CAD build for the part. Positions are in the model's coordinates, mm. A direction names the side the tool comes from. Coordinates: 2 decimals unless noted, no trailing zeros. Loops run counter-clockwise (first coordinate to the right, second up) from the corner with the lowest first, then second, coordinate; pieces in that order, holes last. Notation, with made-up numbers: (56.25, 60.25) -> (65.25, 60.25) arc R21 ccw to (65.25, 73.25) -> close; hole circle Ø7 at (-36.75, -27). An arc over 180 degrees is marked (long way). Write item = value, one per line. Start each with the question number.
(1) Drill centre lines: line 1 (Z direction, x = 3, y = 17.75); line 2 (Y direction, x = 16.5, z = 5); line 3 (Y direction, x = -14.5, z = 6.5). Where is each one in solid material? Low to high. Write a range as from..to.
(2) Band-saw the part on B-B (x = -17.5). Write the cut outline in (y, z), and give its area (3 significant figures).
(3) Pull direction X, two halves, no side cores. Call faces 1 (the face through (-21.5, 20, 0)), 2 (the face through (-16.49, 22.86, 7.39)), 3 (the face through (9, 18.8, 0)): +X half, -X half, draft (parallel to the pull), parting line (faces both ways), or undercut.
(4) Flat gauge pins, fed straight in: P1, Ø15, axis at x = -9.5, y = 5, coming from the -Z side; P2, Ø4, axis at x = 13.5, z = -9, coming from the -Y side; P3, Ø12, axis at x = 12, y = 21, coming from the -Z side; P4, Ø5, axis at y = 14, z = 5.5, coming from the +X side. Where does each tip first touch, or does it go through?
(5) Tool access for faces 4 (the face through (18.51, 22.86, 7.39)), 5 (the face through (-5, 9, -8.5)), 6 (the face through (-16.5, 9, 0)), 7 (the face through (-5, 9, 8)): list every direction of +Z, -Z, +X, -X, +Y, -Y with a clear straight run to the whole face (end or side of a thin tool).
(6) Band-saw the part on C-C (y = 14.75). Write the cut outline in (x, z), and give its area (3 significant figures).
(7) Band-saw the part on D-D (x = 1). Write the cut outline in (y, z).
(8) Band-saw the part on A-A (z = 8.5). Write the cut outline in (x, y), and give its area (3 significant figures).
```python
from build123d import *

# Parameters (mm, degrees)
P01_STANDOFF_START                = 20.4
SK_P01_STANDOFF_R                 = 1.5
P01_STANDOFF_DEPTH                = 5
P02_STANDOFF_START                = 20.4
SK_P02_STANDOFF_R                 = 1.5
P02_STANDOFF_DEPTH                = 5
P03_STANDOFF_START                = 20.4
SK_P03_STANDOFF_R                 = 1.5
P03_STANDOFF_DEPTH                = 5
P04_STANDOFF_START                = 20.4
SK_P04_STANDOFF_R                 = 1.5
P04_STANDOFF_DEPTH                = 5
P05_POLOLURCSWITCHWITHRELAY_START = 18.8
SK_P05_POLOLURCSWITCHWITHRELAY_W  = 43
SK_P05_POLOLURCSWITCHWITHRELAY_H  = 25
P05_POLOLURCSWITCHWITHRELAY_DEPTH = 1.6
SK_P06_RELAYG5LE_W                = 22.5
SK_P06_RELAYG5LE_H                = 16.5
P06_RELAYG5LE_DEPTH               = 18.8


with BuildPart() as part:
    # SK_P01_Standoff → P01_Standoff (new body)
    with BuildSketch(Plane(origin=(0, 0, 0), x_dir=(1, 0, 0), z_dir=(0, 1, 0)).offset(P01_STANDOFF_START)):
        with Locations(Location((-17.5, 8.5, 0), (0, 0, 270))):
            Circle(SK_P01_STANDOFF_R)
    extrude(amount=P01_STANDOFF_DEPTH)



with BuildPart() as body_2:
    # SK_P02_Standoff → P02_Standoff (new body)
    with BuildSketch(Plane(origin=(0, 0, 0), x_dir=(1, 0, 0), z_dir=(0, 1, 0)).offset(P02_STANDOFF_START)):
        with Locations(Location((-17.5, -8.5, 0), (0, 0, 270))):
            Circle(SK_P02_STANDOFF_R)
    extrude(amount=P02_STANDOFF_DEPTH)


with BuildPart() as body_3:
    # SK_P03_Standoff → P03_Standoff (new body)
    with BuildSketch(Plane(origin=(0, 0, 0), x_dir=(1, 0, 0), z_dir=(0, 1, 0)).offset(P03_STANDOFF_START)):
        with Locations(Location((17.5, 8.5, 0), (0, 0, 270))):
            Circle(SK_P03_STANDOFF_R)
    extrude(amount=P03_STANDOFF_DEPTH)


with BuildPart() as body_4:
    # SK_P04_Standoff → P04_Standoff (new body)
    with BuildSketch(Plane(origin=(0, 0, 0), x_dir=(1, 0, 0), z_dir=(0, 1, 0)).offset(P04_STANDOFF_START)):
        with Locations(Location((17.5, -8.5, 0), (0, 0, 270))):
            Circle(SK_P04_STANDOFF_R)
    extrude(amount=P04_STANDOFF_DEPTH)


with BuildPart() as part_1:
    add(part.part)

    add(body_2.part)  # P05_PololuRCswitchwithrelay merges body 2

    add(body_3.part)  # P05_PololuRCswitchwithrelay merges body 3

    add(body_4.part)  # P05_PololuRCswitchwithrelay merges body 4
    # SK_P05_PololuRCswitchwithrelay → P05_PololuRCswitchwithrelay (add)
    with BuildSketch(Plane(origin=(0, 0, 0), x_dir=(1, 0, 0), z_dir=(0, 1, 0)).offset(P05_POLOLURCSWITCHWITHRELAY_START)):
        Rectangle(SK_P05_POLOLURCSWITCHWITHRELAY_W, SK_P05_POLOLURCSWITCHWITHRELAY_H)
    extrude(amount=P05_POLOLURCSWITCHWITHRELAY_DEPTH)

    # SK_P06_RelayG5LE → P06_RelayG5LE (add)
    with BuildSketch(Plane(origin=(0, 0, 0), x_dir=(1, 0, 0), z_dir=(0, 1, 0))):
        with Locations((-5.25, 0.25)):
            Rectangle(SK_P06_RELAYG5LE_W, SK_P06_RELAYG5LE_H)
    extrude(amount=P06_RELAYG5LE_DEPTH)


solid = part_1.part
```
Findings below:
q1.line_1 = -8.5..8
q1.line_2 = 18.8..20.4
q1.line_3 = 0..20.4
q2.outline = (18.8, -12.5) -> (20.4, -12.5) -> (20.4, -10) -> (25.4, -10) -> (25.4, -7) -> (20.4, -7) -> (20.4, 7) -> (25.4, 7) -> (25.4, 10) -> (20.4, 10) -> (20.4, 12.5) -> (18.8, 12.5) -> close
q2.area = 70.0 mm²
q3.face_1 = -X half
q3.face_2 = undercut
q3.face_3 = draft
q4.P1 = -8.5
q4.P2 = 18.8
q4.P3 = -12.5
q4.P4 = 6
q5.face_4 = +Y
q5.face_5 = -Z, +X, -X, -Y
q5.face_6 = +Z, -Z, -X, -Y
q5.face_7 = +Z, +X, -X, -Y
q6.outline = (-16.5, -8.5) -> (6, -8.5) -> (6, 8) -> (-16.5, 8) -> close
q6.area = 371 mm²
q7.outline = (0, -8.5) -> (18.8, -8.5) -> (18.8, -12.5) -> (20.4, -12.5) -> (20.4, 12.5) -> (18.8, 12.5) -> (18.8, 8) -> (0, 8) -> close
q8.outline = (-21.5, 18.8) -> (21.5, 18.8) -> (21.5, 20.4) -> (19, 20.4) -> (19, 25.4) -> (16, 25.4) -> (16, 20.4) -> (-16, 20.4) -> (-16, 25.4) -> (-19, 25.4) -> (-19, 20.4) -> (-21.5, 20.4) -> close
q8.area = 98.8 mm²
